```python
from build123d import *

# Parameters (mm, degrees)
BOSS_EXTRUDE1_DEPTH = 2
BOSS_EXTRUDE2_DEPTH = 8
SKETCH3_W           = 22.1
SKETCH3_H           = 30
BOSS_EXTRUDE3_DEPTH = 20
BOSS_EXTRUDE3_TAPER = 9


with BuildPart() as part:
    # Sketch1 → Boss-Extrude1 (new body)
    with BuildSketch(Plane.XY):
        with BuildLine():
            Line((-10.5, -15.75), (10.5, -15.75))
            ThreePointArc((10.5, -15.75), (11.914213562, -15.164213562), (12.5, -13.75))
            Line((12.5, -13.75), (12.5, 13.75))
            ThreePointArc((12.5, 13.75), (11.914213562, 15.164213562), (10.5, 15.75))
            Line((10.5, 15.75), (-10.5, 15.75))
            ThreePointArc((-10.5, 15.75), (-11.914213562, 15.164213562), (-12.5, 13.75))
            Line((-12.5, 13.75), (-12.5, -13.75))
            ThreePointArc((-12.5, -13.75), (-11.914213562, -15.164213562), (-10.5, -15.75))
        make_face()
    extrude(amount=BOSS_EXTRUDE1_DEPTH)

    # Sketch2 → Boss-Extrude2 (add, symmetric)
    with BuildSketch(Plane(origin=(0, 0, 0), x_dir=(0, 0, -1), z_dir=(1, 0, 0))):
        with BuildLine():
            Line((-2, 12.000372018), (-2, -12.000372018))
            ThreePointArc((-2, -12.000372018), (-4.886867761, -11.141250022), (-7.474198634, -9.599233477))
            ThreePointArc((-7.474198634, -9.599233477), (-7.810172539, -9.12144706), (-7.821933208, -8.537477873))
            Line((-7.821933208, -8.537477873), (-2, 12.000372018))
        make_face()
    extrude(amount=BOSS_EXTRUDE2_DEPTH, both=True)

    # Sketch3 → Boss-Extrude3 (add)
    with BuildSketch(Plane(origin=(0, 0, 0), x_dir=(-1, 0, 0), z_dir=(0, 0, -1))):
        Rectangle(SKETCH3_W, SKETCH3_H)
    extrude(amount=BOSS_EXTRUDE3_DEPTH, taper=BOSS_EXTRUDE3_TAPER)


solid = part.part
```
The listing builds one solid part. Answer for the finished solid, in the listing's coordinates (mm). A direction names the side the tool comes from. Coordinates: 2 decimals unless noted, no trailing zeros. Return JSON: item names as keys, results as strings. Group by question number.
1. Straight lines are drawn through the part: L1, parallel to X at y = -5, z = 5.75; L2, parallel to X at y = 0, z = -3.5; L3, parallel to Z at x = 1, y = 9.5. For each, find the intervals that lie inside material, in ascending order.
2. Which of the six approach directions +Z, -Z, +X, -X, +Y, -Y give full straight-line access (tool end or side, diameter ignored) to faces 1 (the flat face through (8, -2, 4)), 2 (the cylindrical face through (11.93, 15.15, 0.99)), 3 (the flat face through (-8, -2, 4))?
3. Given pin 1 (6 mm diameter, centred on x = -9, y = -11, fed in from -Z); pin 2 (8 mm diameter, centred on x = -9.5, z = -6, fed in from +Y); pin 3 (10 mm diameter, centred on x = 8.5, z = -14.5, fed in from +Y); pin 4 (8 mm diameter, centred on x = -5.5, y = 4.5, fed in from +Z), each flat-ended and moving along its own axis, determine where each tip first touches the part or whether it passes through.
Ans:
{
 "1": {"L1": "-8 to 8", "L2": "-10.5 to 10.5", "L3": "-20 to 2.71"},
 "2": {"face 1": "+Z, +X, +Y, -Y", "face 2": "+Z, -Z, +X, +Y", "face 3": "+Z, -X, +Y, -Y"},
 "3": {"pin 1": "z = -20", "pin 2": "y = 14.68", "pin 3": "y = 13.5", "pin 4": "z = 5.26"}
}
